Geometry: see drawing. Coordinates: mm, zero at the bounding-box minimum. A direction names the side the tool comes from. Round coordinates to 2 decimals unless told otherwise and drop trailing zeros. Loops run counter-clockwise (first coordinate to the right, second up) from the corner with the lowest first, then second, coordinate; pieces in that order, holes last.
(1) Material intervals for probe 1 along Y at (x, z) = (1.55, 5.15); probe 2 along Y at (x, z) = (2.8, 5.6) (1 decimal); probe 3 along Y at (x, z) = (3.2, 3.55) (1 decimal), sorted ascending.
(2) Mould query, pull axis Y, two halves, no side actions, for the marked faces 1, 2 and 3. Classes: pulls with the +Y half, pulls with the -Y half, needs draft (parallel to the pull), parting line crosses it, or undercut.
(3) First-contact query: pin 1 Ø1 at (x, z) = (3.5, 5) entering from -Y; pin 2 Ø3 at (x, z) = (1, 3) entering from -Y; pin 3 Ø0.9 at (x, z) = (2, 5.5) entering from +Y. Flat tips, straight axial feed; report the tip coordinate or a pass-through.
(4) Section B-B, the plane y = 2.8. Return the cut outline in (x, z).
(5) Section C-C, the plane z = 2.3. Return the cut outline in (x, y).
(6) Set-up query: the marked faces 4 and 5. Return all of +Z, -Z, +X, -X, +Y, -Y with unobstructed straight access to the full face (end or side cutting, diameter ignored); none if empty.
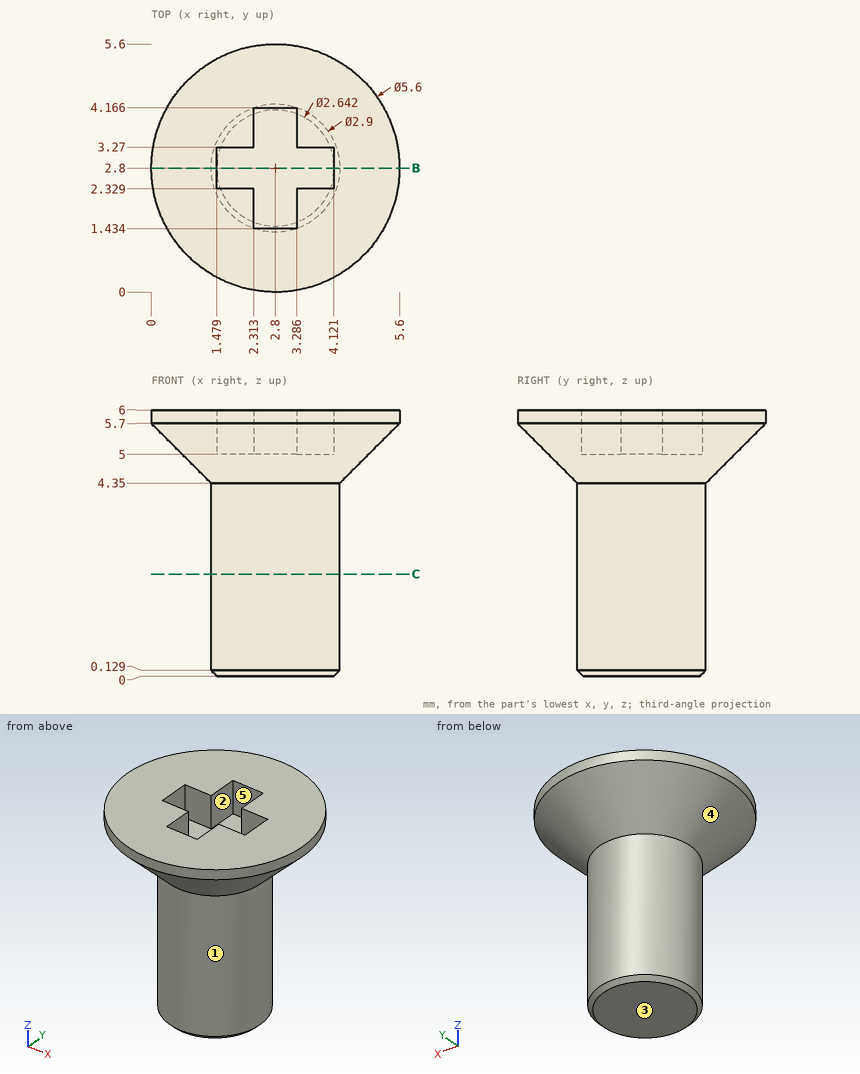
Output values:
1. probe 1: y = 0.93 to 2.33, 3.27 to 4.67
1. probe 2: y = 0.1 to 1.4, 4.2 to 5.5
1. probe 3: y = 1.4 to 4.2
2. face 1: parting line crosses it
2. face 2: undercut
2. face 3: needs draft
3. pin 1: stops at y = 0.28
3. pin 2: stops at y = 1.38
3. pin 3: stops at y = 5.57
4. outline: (0, 5.7) - (1.35, 4.35) - (1.35, 0.13) - (1.48, 0) - (4.12, 0) - (4.25, 0.13) - (4.25, 4.35) - (5.6, 5.7) - (5.6, 6) - (4.12, 6) - (4.12, 5) - (1.48, 5) - (1.48, 6) - (0, 6) - close
5. outline: circle Ø2.9 at (2.8, 2.8)
6. face 4: -Z
6. face 5: +Z
